Check sheet for the modelled part. Datum: model origin and axes. Units: mm. A direction names the side the tool comes from. Give positions to 0.01 mm unless a question says otherwise; leave off trailing zeros. Order: outer loops, then holes, each group sorted by start corner. A loop starts at its lowest first (then second) coordinate and runs counter-clockwise, first axis right, second up.
Item 1: Sectioned sample at D-D on z = -17. Record the boundary of the cut face in (x, y), and give its area (3 significant figures).
Item 2: Sectioned sample at B-B on z = -1. Record the boundary of the cut face in (x, y).
Item 3: Sectioned sample at A-A on x = 0. Record the boundary of the cut face in (y, z).
Item 4: Access from +Z, -Z, +X, -X, +Y, -Y to the whole of each face (thin tool, end or side, straight path). Record for faces 1 (the cylindrical face through (-8.75, 0.05, -7.4)), 2 (the flat face through (1, 1, -43.2)), 3 (the flat face through (0, -7.7, -28)).
Item 5: Sectioned sample at C-C on y = 0. Record the boundary of the cut face in (x, z).
Item 6: Release check for a two-part mould opening along X. For faces 4 (the cylindrical face through (3.233, -1.341, 1.479)), 5 (the flat face through (8, 0, -15)), 6 (the flat face through (0, 0, -49.2)) record: released by +X, released by -X, zero draft, split by the parting line, or undercut.
Item 7: Gauge pin test, flat ends, axial feed: P1, Ø1.8, axis at x = 1, y = 9.5, coming from the -Z side; P2, Ø3, axis at x = -7.5, y = 0, coming from the +Z side; P3, Ø1, axis at x = 6.5, z = -26, coming from the -Y side; P4, Ø1, axis at x = 7, y = 8, coming from the +Z side. Record the tip position at first contact, or that the pin passes through.
Item 8: Material ranges on line 1 along Y through (x, z) = (-4, -23); line 2 along Z through (x, y) = (3.5, 3.75); line 3 along Z through (x, y) = (-7.5, -1), recorded low to high.
from build123d import *

# Parameters (mm, degrees)
SKETCH1_R               = 10
BOSS_EXTRUDE1_DEPTH     = 41.1
SKETCH2_W               = 25.1
SKETCH2_H               = 2.3
CUT_EXTRUDE1_DEPTH      = 44.465043426
SKETCH3_R               = 3.5
BOSS_EXTRUDE2_DEPTH     = 3
SKETCH5_R               = 2
BOSS_EXTRUDE4_DEPTH     = 14.5
CUT_EXTRUDE2_DEPTH      = 44.465043426
CUT_EXTRUDE2_DEPTH_BACK = 44.465043426
SKETCH6_W               = 14.5
SKETCH6_H               = 0.5
SKETCH7_R               = 3.1
BOSS_EXTRUDE5_DEPTH     = 2.1
SKETCH8_R               = 1
BOSS_EXTRUDE6_DEPTH     = 6
SKETCH10_R              = 1.25
CUT_EXTRUDE3_DEPTH      = 15


with BuildPart() as part:
    # Sketch1 → Boss-Extrude1 (new body)
    with BuildSketch(Plane.XY):
        Circle(SKETCH1_R)
    extrude(amount=-BOSS_EXTRUDE1_DEPTH)

    # Sketch2 → Cut-Extrude1 (cut, symmetric)
    with BuildSketch(Plane(origin=(0, 0, 0), x_dir=(0, 0, -1), z_dir=(1, 0, 0))):
        with Locations((28.55, 8.85)):
            Rectangle(SKETCH2_W, SKETCH2_H)
    cut_extrude1 = extrude(amount=CUT_EXTRUDE1_DEPTH, both=True, mode=Mode.SUBTRACT)

    # Mirror1: Cut-Extrude1 across plane
    add(cut_extrude1.mirror(Plane.ZX), mode=Mode.SUBTRACT)

    # Sketch3 → Boss-Extrude2 (add)
    with BuildSketch(Plane.XY):
        Circle(SKETCH3_R)
    extrude(amount=BOSS_EXTRUDE2_DEPTH)

    # Sketch5 → Boss-Extrude4 (add)
    with BuildSketch(Plane.XY.offset(3)):
        with Locations(Location((0, 0, 0), (0, 0, 180))):
            Circle(SKETCH5_R)
    extrude(amount=BOSS_EXTRUDE4_DEPTH)

    # Sketch6 → Cut-Extrude2 (cut, two sides: drawn at the far end of the back side and taken through both)
    with BuildSketch(Plane(origin=(0, 0, 0), x_dir=(0, 0, -1), z_dir=(1, 0, 0)).offset(-CUT_EXTRUDE2_DEPTH_BACK)):
        with Locations((-10.25, 1.75)):
            Rectangle(SKETCH6_W, SKETCH6_H)
    extrude(amount=CUT_EXTRUDE2_DEPTH + CUT_EXTRUDE2_DEPTH_BACK, mode=Mode.SUBTRACT)

    # Sketch7 → Boss-Extrude5 (add)
    with BuildSketch(Plane(origin=(0, 0, -41.1), x_dir=(-1, 0, 0), z_dir=(0, 0, -1))):
        Circle(SKETCH7_R)
    extrude(amount=BOSS_EXTRUDE5_DEPTH)

    # Sketch8 → Boss-Extrude6 (add)
    with BuildSketch(Plane(origin=(0, 0, -43.2), x_dir=(-1, 0, 0), z_dir=(0, 0, -1))):
        Circle(SKETCH8_R)
    extrude(amount=BOSS_EXTRUDE6_DEPTH)

    # Sketch10 → Cut-Extrude3 (cut)
    with BuildSketch(Plane.XY):
        with Locations((-7.5, 0)):
            Circle(SKETCH10_R)
    cut_extrude3 = extrude(amount=-CUT_EXTRUDE3_DEPTH, mode=Mode.SUBTRACT)

    # Mirror2: Cut-Extrude3 across plane
    add(cut_extrude3.mirror(Plane(origin=(0, 0, 0), x_dir=(0, 0, 1), z_dir=(1, 0, 0))), mode=Mode.SUBTRACT)


solid = part.part
Report:
1. outline: (-6.38, -7.7) - (6.38, -7.7) arc R10 ccw to (6.38, 7.7) - (-6.38, 7.7) arc R10 ccw to start
1. area: 274 mm2
2. outline: circle Ø20 at (0, 0); hole circle Ø2.5 at (-7.5, 0); hole circle Ø2.5 at (7.5, 0)
3. outline: (-10, -16) - (-7.7, -16) - (-7.7, -41.1) - (-3.1, -41.1) - (-3.1, -43.2) - (-1, -43.2) - (-1, -49.2) - (1, -49.2) - (1, -43.2) - (3.1, -43.2) - (3.1, -41.1) - (7.7, -41.1) - (7.7, -16) - (10, -16) - (10, 0) - (3.5, 0) - (3.5, 3) - (1.5, 3) - (1.5, 17.5) - (-2, 17.5) - (-2, 3) - (-3.5, 3) - (-3.5, 0) - (-10, 0) - close
4. face 1: +Z
4. face 2: -Z
4. face 3: -Z, +X, -X, -Y
5. outline: (-10, -41.1) - (-3.1, -41.1) - (-3.1, -43.2) - (-1, -43.2) - (-1, -49.2) - (1, -49.2) - (1, -43.2) - (3.1, -43.2) - (3.1, -41.1) - (10, -41.1) - (10, 0) - (8.75, 0) - (8.75, -15) - (6.25, -15) - (6.25, 0) - (3.5, 0) - (3.5, 3) - (2, 3) - (2, 17.5) - (-2, 17.5) - (-2, 3) - (-3.5, 3) - (-3.5, 0) - (-6.25, 0) - (-6.25, -15) - (-8.75, -15) - (-8.75, 0) - (-10, 0) - close
6. face 4: split by the parting line
6. face 5: undercut
6. face 6: zero draft
7. P1: stops at z = -16
7. P2: stops at z = 0
7. P3: stops at y = -7.7
7. P4: passes through
8. line 1: y = -7.7 to 7.7
8. line 2: z = -41.1 to 0
8. line 3: z = -41.1 to -15
